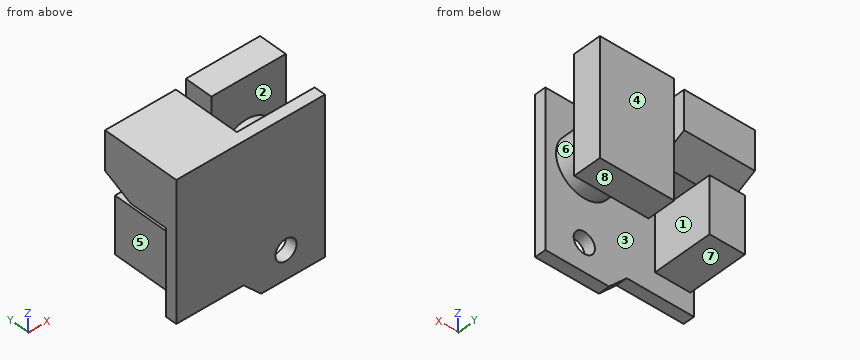
```python
from build123d import *

# Parameters (mm, degrees)
SKETCH1_W           = 21
SKETCH1_H           = 22
BOSS_EXTRUDE1_DEPTH = 1.6
SKETCH2_R           = 1.5
CUT_EXTRUDE1_DEPTH  = 1.6
SKETCH3_W           = 5
SKETCH3_H           = 8
BOSS_EXTRUDE2_DEPTH = 8.5
SKETCH4_W           = 10
SKETCH4_H           = 7.5
BOSS_EXTRUDE3_DEPTH = 9.5
CHAMFER1_SIZE       = 4
CHAMFER1_SIZE2      = 2
SKETCH5_R           = 4
BOSS_EXTRUDE4_DEPTH = 4.5
SKETCH6_W           = 10.5
SKETCH6_H           = 16.5
BOSS_EXTRUDE5_DEPTH = 4


with BuildPart() as part:
    # Sketch1 → Boss-Extrude1 (new body)
    with BuildSketch(Plane(origin=(0, 0, 0), x_dir=(1, 0, 0), z_dir=(0, 1, 0))):
        Rectangle(SKETCH1_W, SKETCH1_H)
    extrude(amount=BOSS_EXTRUDE1_DEPTH)

    # Sketch2 → Cut-Extrude1 (cut)
    with BuildSketch(Plane(origin=(0, 1.6, 0), x_dir=(1, 0, 0), z_dir=(0, 1, 0))):
        with Locations(Location((5, 7, 0), (0, 0, 270))):
            Circle(SKETCH2_R)
        Polygon((-12.078029191, 8.5), (-1, 8.5), (1.5, 11), (-12.078029191, 11), align=None)
    extrude(amount=-CUT_EXTRUDE1_DEPTH, mode=Mode.SUBTRACT)

    # Sketch3 → Boss-Extrude2 (add)
    with BuildSketch(Plane(origin=(0, 1.6, 0), x_dir=(1, 0, 0), z_dir=(0, 1, 0))):
        with Locations((-7.5, 1.5)):
            Rectangle(SKETCH3_W, SKETCH3_H)
    extrude(amount=BOSS_EXTRUDE2_DEPTH)

    # Sketch4 → Boss-Extrude3 (add)
    with BuildSketch(Plane(origin=(0, 1.6, 0), x_dir=(1, 0, 0), z_dir=(0, 1, 0))):
        with Locations((-5.5, -7.25)):
            Rectangle(SKETCH4_W, SKETCH4_H)
    extrude(amount=BOSS_EXTRUDE3_DEPTH)

    # Chamfer1
    chamfer1_edges = [part.edges().sort_by_distance(p)[0] for p in [
        (-5.5, 11.1, 3.5),
    ]]
    chamfer1_side = [part.faces().sort_by_distance(p)[0] for p in [
        (-5.5, 6.35, 3.5),
    ]]
    chamfer(chamfer1_edges, length=CHAMFER1_SIZE, length2=CHAMFER1_SIZE2, reference=chamfer1_side[0])

    # Sketch5 → Boss-Extrude4 (add)
    with BuildSketch(Plane(origin=(0, 1.6, 0), x_dir=(1, 0, 0), z_dir=(0, 1, 0))):
        with Locations(Location((5, -3, 0), (0, 0, 270))):
            Circle(SKETCH5_R)
    extrude(amount=BOSS_EXTRUDE4_DEPTH)

    # Sketch6 → Boss-Extrude5 (add)
    with BuildSketch(Plane(origin=(0, 6.1, 0), x_dir=(1, 0, 0), z_dir=(0, 1, 0))):
        with Locations((5.25, -4.55)):
            Rectangle(SKETCH6_W, SKETCH6_H)
    extrude(amount=BOSS_EXTRUDE5_DEPTH)


solid = part.part
```
CAD build for the part. Positions are in the model's coordinates, mm. Face numbers are marked on the shaded views. A direction names the side the tool comes from. Give positions to 0.01 mm unless a question says otherwise; leave off trailing zeros. Write each loop counter-clockwise with the first axis right and the second up, starting at its lowest first coordinate (ties: lowest second). Pieces come first, ordered by that corner, then holes. Notation, with made-up numbers: M 3,27 L 24,27 A21 ccw 24,36 Z; hole C 86,53.5 d5. An arc over 180 degrees is marked long. Return JSON: item names as keys, results as strings. Group by question number.
(1) Band-saw the part on C-C (x = 5). Give the cut face in (y, z), and give its area (3 significant figures).
(2) 3-axis set-ups, long thin cutter, end or side, ignore diameter. For the marked faces 5, 6, 7 and 8: which of +Z, -Z, +X, -X, +Y, -Y reach the whole face in a straight line?
(3) Flat gauge pins, fed straight in: pin 1 Ø2.5 at (x, y) = (-7, 7) entering from -Z; pin 2 Ø4.5 at (x, y) = (5.5, 8) entering from -Z; pin 3 Ø0.5 at (x, y) = (-7, 1) entering from -Z. Where does each tip first touch, or does it go through?
(4) Drill centre lines: L1, parallel to Z at x = -8, y = 5.75; L2, parallel to Y at x = 6.5, z = -3; L3, parallel to Z at x = 2.25, y = 9.75. Where is each one in solid material? Low to high. Write a range as [from, to].
(5) Band-saw the part on A-A (y = 3.5). Give the cut face in (x, z), and give its area (3 significant figures).
(6) Band-saw the part on B-B (z = -7). Give the cut face in (x, y), and give its area (3 significant figures).
(7) Mould opens along Y. For the marked faces 1, 2, 3 and 4 say: pulls with the +Y half, pulls with the -Y half, needs draft (parallel to the pull), parting line crosses it, or undercut.
(8) Band-saw the part on D-D (z = 3). Give the cut face in (x, y), and give its area (3 significant figures).
Entries:
{
 "1": {"outline": "M 0,-11 L 1.6,-11 L 1.6,-8.5 L 0,-8.5 Z; M 0,-5.5 L 1.6,-5.5 L 1.6,-1 L 6.1,-1 L 6.1,-3.7 L 10.1,-3.7 L 10.1,12.8 L 6.1,12.8 L 6.1,7 L 1.6,7 L 1.6,11 L 0,11 Z", "area": "132 mm^2"},
 "2": {"face 5": "-Z, -X, +Y", "face 6": "none", "face 7": "-Z, +X, -X, +Y", "face 8": "-Z, +X, +Y"},
 "3": {"pin 1": "stops at z = -5.5", "pin 2": "stops at z = -3.7", "pin 3": "stops at z = -8.5"},
 "4": {"L1": "z = [-5.5, 2.5], [3.5, 11]", "L2": "y = [0, 1.6], [6.1, 10.1]", "L3": "z = [-3.7, 12.8]"},
 "5": {"outline": "M -10.5,3.5 L -0.5,3.5 L -0.5,11 L -10.5,11 Z; M -10,-5.5 L -5,-5.5 L -5,2.5 L -10,2.5 Z; C 5,3 d8", "area": "165 mm^2"},
 "6": {"outline": "M -10.5,0 L 3.5,0 L 3.5,1.6 L -10.5,1.6 Z; M 6.5,0 L 10.5,0 L 10.5,1.6 L 6.5,1.6 Z", "area": "28.8 mm^2"},
 "7": {"face 1": "needs draft", "face 2": "undercut", "face 3": "undercut", "face 4": "pulls with the +Y half"},
 "8": {"outline": "M -10.5,0 L 10.5,0 L 10.5,1.6 L 9,1.6 L 9,6.1 L 10.5,6.1 L 10.5,10.1 L 0,10.1 L 0,6.1 L 1,6.1 L 1,1.6 L -10.5,1.6 Z", "area": "112 mm^2"}
}
